CAD build for the part. Positions are in the model's coordinates, mm. A direction names the side the tool comes from. Coordinates: 2 decimals unless noted, no trailing zeros. Write each loop counter-clockwise with the first axis right and the second up, starting at its lowest first coordinate (ties: lowest second). Pieces come first, ordered by that corner, then holes. Notation, with made-up numbers: (2.25, 15) -> (14.25, 15) arc R20 cw to (14.25, 53) -> close; hole circle Ø7 at (33, 42). An arc over 180 degrees is marked (long way). Answer as CSV lines item,"result".
Solid Edge part; units mm, degrees
sketch "Sketch1" plane through (0, 0, 0) normal (0, -1, 0) x (1, 0, 0)
  line L0 (40, 59) -> (0, 59)
  line L1 (0, 59) -> (0, 0)
  line L2 (0, 0) -> (40, 0)
  line L3 (40, 0) -> (40, 14.5)
  line L4 (40, 14.5) -> (10, 14.5)
  line L5 (10, 14.5) -> (10, 44.5)
  line L6 (10, 44.5) -> (40, 44.5)
  line L7 (40, 44.5) -> (40, 59)
extrude "Protrusion1" add sketch "Sketch1" against normal blind 10
hole "Furo_1" at (19.9157, 0, 51.7514) direction (0, 1, 0) diameter 5 end up to next counterbore diameter 9 counterbore depth 5
hole "Hole1" at (20, 0, 7.25) direction (0, 1, 0) diameter 5 end up to next counterbore diameter 9 counterbore depth 5
hole "Furo_3" at (8, 5, 0) direction (0, 0, 1) diameter 3.3 depth 10 tip angle 118
hole "Furo_4" at (32, 5, 0) direction (0, 0, 1) diameter 3.3 depth 10 tip angle 118
hole "Furo_5" at (32, 5, 59) direction (0, 0, -1) diameter 3.3 depth 10 tip angle 118
hole "Hole2" at (8, 5, 59) direction (0, 0, -1) diameter 3.3 depth 10 tip angle 118
hole "Furo_7" at (0, 5, 53.5) direction (1, 0, 0) diameter 1.6 depth 5.2 tip angle 118
hole "Hole3" at (0, 5, 5.5) direction (1, 0, 0) diameter 1.6 depth 5.2 tip angle 118
Item 1: Saw through at A-A on z = 7.25. Give the cut face in (x, y), and give its area (3 significant figures).
Answer below:
outline,"(0, 0) -> (15.5, 0) -> (15.5, 5) -> (17.5, 5) -> (17.5, 10) -> (0, 10) -> close; (22.5, 5) -> (24.5, 5) -> (24.5, 0) -> (40, 0) -> (40, 10) -> (22.5, 10) -> close; hole circle Ø3.3 at (8, 5); hole circle Ø3.3 at (32, 5)"
area,"313 mm2"
Item 2: 3-axis set-ups, long thin cutter, end or side, ignore diameter. For faces 4 (the cylindrical face through (30.364, 4.785, 5.07)), 5 (the cylindrical face through (2.6, 5, 52.7)), 6 (the cylindrical face through (19.718, 2.535, 56.247)): which of +Z, -Z, +X, -X, +Y, -Y reach the whole face in a straight line?
Answer below:
face 4,"-Z"
face 5,"-X"
face 6,"-Y"
Item 3: Wall check: line 1 (Z direction, x = 20, y = 6.45); line 2 (Z direction, x = 3, y = 5); line 3 (Z direction, x = 35.5, y = 5). Give the ranges that are in metal, low to high. Write a range as from..to.
Answer below:
line 1,"z = 0..4.75, 9.75..14.5, 44.5..49.25, 54.25..59"
line 2,"z = 0..4.7, 6.3..52.7, 54.3..59"
line 3,"z = 0..14.5, 44.5..59"
Item 4: Two-plate mould, pull along X, no slides. Class faces 1 (the conical face through (5.597, 4.947, 53.628)), 2 (the cylindrical face through (30.364, 5.215, 53.93)), 3 (the flat face through (7, 0, 30)): pulls with the +X half, pulls with the -X half, needs draft (parallel to the pull), parting line crosses it, or undercut.
Answer below:
face 1,"pulls with the -X half"
face 2,"undercut"
face 3,"needs draft"
Item 5: Saw through at C-C on z = 23.5. Give the cut face in (x, y).
Answer below:
outline,"(0, 0) -> (10, 0) -> (10, 10) -> (0, 10) -> close"
Item 6: Flat gauge pins, fed straight in: pin 1 (1 mm diameter, centred on y = 5, z = 53.5, fed in from -X); pin 2 (1 mm diameter, centred on y = 6, z = 22, fed in from +X); pin 3 (6.5 mm diameter, centred on x = 20, z = 7.25, fed in from -Y). Where does each tip first touch, or does it go through?
Answer below:
pin 1,"stops at x = 5.38"
pin 2,"stops at x = 10"
pin 3,"stops at y = 5"
Item 7: Saw through at B-B on x = 34.5. Give the cut face in (y, z).
Answer below:
outline,"(0, 0) -> (10, 0) -> (10, 14.5) -> (0, 14.5) -> close; (0, 44.5) -> (10, 44.5) -> (10, 59) -> (0, 59) -> close"
